Read the model definition and answer for the solid it produces. Units are mm, in the model's axes. A direction names the side the tool comes from. Coordinates: 2 decimals unless noted, no trailing zeros. Write each loop counter-clockwise with the first axis right and the second up, starting at its lowest first coordinate (ties: lowest second). Pieces come first, ordered by that corner, then holes. Notation, with made-up numbers: (-3.75, 18) -> (38.25, 18) arc R23 ccw to (38.25, 26) -> close; hole circle Ø4 at (-32.75, -8). An arc over 180 degrees is marked (long way). One line per item, written item: value. Start each with the question number.
1. For faces 1 (the flat face through (-1, 0, -50)), 2 (the flat face through (1, 4.536, 22)), determine the directions among +Z, -Z, +X, -X, +Y, -Y from which every point of the face is accessible in a straight line to the end or side of a thin tool.
2. Find section A-A, the plane x = -17. Write down the section's boundary in (y, z).
3. Given P1, Ø16, axis at x = -12, y = 11.5, coming from the +Z side; P2, Ø12, axis at x = 6.5, z = 7, coming from the +Y side; P3, Ø10, axis at x = -38.5, y = 7, coming from the +Z side, each flat-ended and moving along its own axis, determine where each tip first touches the part or whether it passes through.
4. Consider line 1 along Y through (x, z) = (19, 35); line 2 along Z through (x, y) = (29.5, 12.5); line 3 along Z through (x, y) = (-11.5, 0.5). Determine where each line is inside the solid, lowest interval first.
5. Find section B-B, the plane z = 34. Write down the section's boundary in (x, y), and give its area (3 significant figures).
6. Find section C-C, the plane y = 16. Write down the section's boundary in (x, z).
```python
from build123d import *

# Parameters (mm, degrees)
F0_W     = 112.5419810414
F0_H     = 49.071829766
F1_DEPTH = 50
F2_DEPTH = 50
F3_W     = 112.5419810414
F3_H     = 5.3821941838
F3_H_2   = 46.7423561029
F4_DEPTH = 20
F5_R     = 5


with BuildPart() as f1:
    # F0 (on Top) → F1 (new body)
    with BuildSketch(Plane.XY):
        Rectangle(F0_W, F0_H)
    extrude(amount=F1_DEPTH)

    # F2 (add): a face of the model
    f2_faces = [f1.faces().sort_by_distance(p)[0] for p in [
        (0, 0, 0),
    ]]
    extrude(f2_faces, amount=F2_DEPTH)

    # F3 (on face) → F4 (cut)
    with BuildSketch(Plane(origin=(0, 24.535914883, 0), x_dir=(-1, 0, 0), z_dir=(0, 1, 0))):
        with Locations((0, 0.5665468052)):
            Rectangle(F3_W, F3_H)
        with Locations((0, 26.6288219485)):
            Rectangle(F3_W, F3_H_2)
    extrude(amount=-F4_DEPTH, mode=Mode.SUBTRACT)

    # F5
    f5_edges = [f1.edges().sort_by_distance(p)[0] for p in [
        (0, 4.535915, 50),
        (-56.270991, -10, 50),
        (56.270991, -24.535915, 0),
        (-56.270991, -24.535915, 0),
    ]]
    fillet(f5_edges, radius=F5_R)


solid = f1.part
```
Answer block:
1. face 1: -Z, +X, -X, +Y, -Y
1. face 2: +Z, +X, -X, +Y
2. outline: (-24.54, -50) -> (24.54, -50) -> (24.54, -2.12) -> (4.54, -2.12) -> (4.54, 45) arc R5 ccw to (-0.46, 50) -> (-24.54, 50) -> close
3. P1: stops at z = 48.05
3. P2: stops at y = 4.54
3. P3: stops at z = 49.35
4. line 1: y = -24.54 to 4.54
4. line 2: z = -50 to -2.12
4. line 3: z = -50 to 49.91
5. outline: (-56.27, -19.54) arc R5 ccw to (-51.27, -24.54) -> (51.27, -24.54) arc R5 ccw to (56.27, -19.54) -> (56.27, 4.54) -> (-56.27, 4.54) -> close
5. area: 3,260 mm2
6. outline: (-56.27, -50) -> (56.27, -50) -> (56.27, -2.12) -> (-56.27, -2.12) -> close
